The figure shows three views and two pictorial views of one solid part (mm, origin at its lowest corner). Answer the questions. A direction names the side the tool comes from. Coordinates: 2 decimals unless noted, no trailing zeros. Order: outer loops, then holes, each group sorted by start corner. A loop starts at its lowest first (then second) coordinate and runs counter-clockwise, first axis right, second up. Notation, with made-up numbers: (30, 45.5) -> (78, 45.5) arc R3 cw to (78, 49.5) -> close; hole circle Ø4 at (47.5, 79). An arc over 180 degrees is marked (long way). Write item = value, one per line.
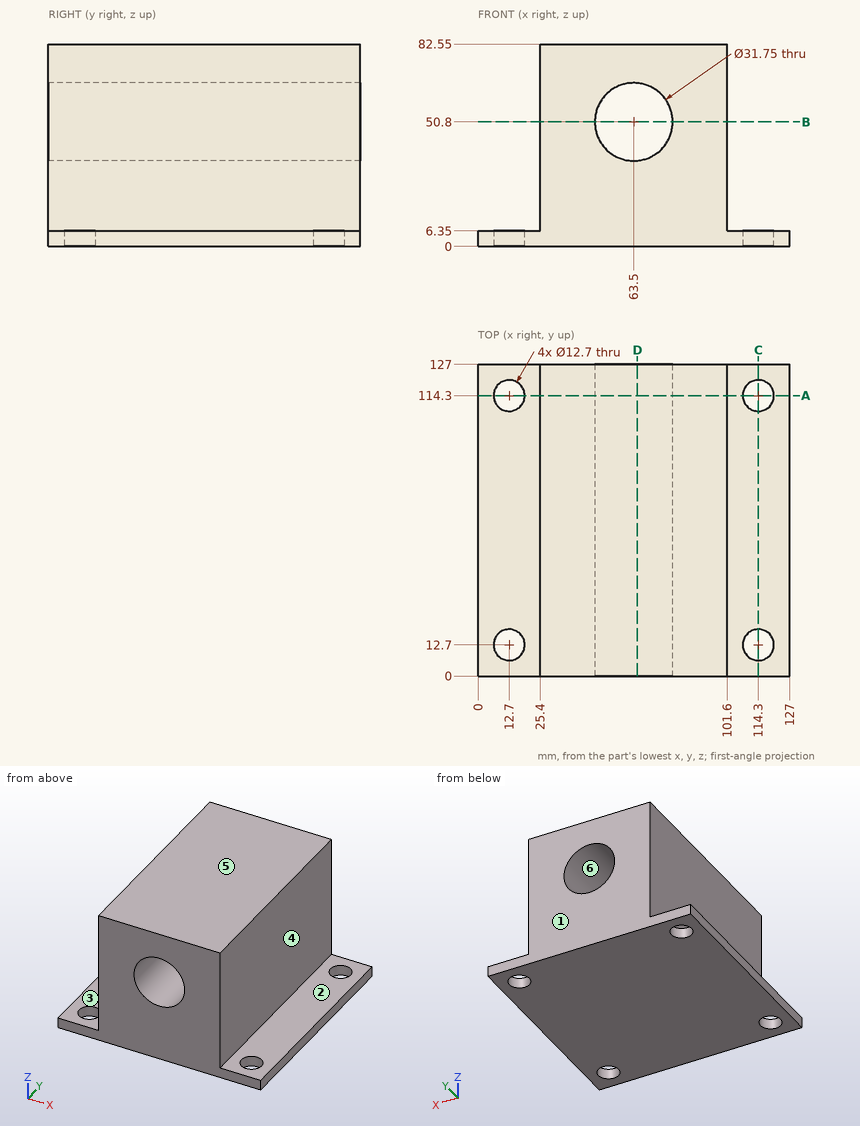
Q1. The mould has two halves that part along X. Classify the marked faces 4, 5 and 6: released by +X, released by -X, zero draft, split by the parting line, or undercut.
The answers:
face_4 = released by +X
face_5 = zero draft
face_6 = undercut
Q2. Section C-C, the plane x = 114.3 is taken. Give the vertices of the cut face in (y, z).
The answers:
outline = (0, 0) -> (6.35, 0) -> (6.35, 6.35) -> (0, 6.35) -> close; (19.05, 0) -> (107.95, 0) -> (107.95, 6.35) -> (19.05, 6.35) -> close; (120.65, 0) -> (127, 0) -> (127, 6.35) -> (120.65, 6.35) -> close
Q3. Section A-A, the plane y = 114.3 is taken. Give the vertices of the cut face in (x, z) (3 decimals).
The answers:
outline = (0, 0) -> (6.35, 0) -> (6.35, 6.35) -> (0, 6.35) -> close; (19.05, 0) -> (107.95, 0) -> (107.95, 6.35) -> (101.6, 6.35) -> (101.6, 82.55) -> (25.4, 82.55) -> (25.4, 6.35) -> (19.05, 6.35) -> close; (120.65, 0) -> (127, 0) -> (127, 6.35) -> (120.65, 6.35) -> close; hole circle Ø31.75 at (63.5, 50.8)
Q4. Section D-D, the plane x = 65 is taken. Give the vertices of the cut face in (y, z).
The answers:
outline = (0, 0) -> (127, 0) -> (127, 35) -> (0, 35) -> close; (0, 66.6) -> (127, 66.6) -> (127, 82.55) -> (0, 82.55) -> close
Q5. Each of these flat-tipped pins is pushed along its axis until it touches: pin 1 Ø3 at (y, z) = (52, 26) entering from +X; pin 2 Ø20.5 at (x, y) = (10.5, 84) entering from +Z; pin 3 Ø3 at (x, y) = (113.5, 96) entering from +Z. Where does it stop, or does it pass through?
The answers:
pin_1 = 101.6
pin_2 = 6.35
pin_3 = 6.35
Q6. Find the intervals of material crossed by line 1 along Y through (x, z) = (12.7, 1.75); line 2 along X through (y, z) = (12, 2); line 3 along X through (y, z) = (59, 50), in increasing order.
The answers:
line_1 = 0 to 6.35, 19.05 to 107.95, 120.65 to 127
line_2 = 0 to 6.39, 19.01 to 107.99, 120.61 to 127
line_3 = 25.4 to 47.65, 79.35 to 101.6
Q7. A tool of negligible diameter and unlimited length cuts with its end or side. For the marked faces 1, 2 and 3, from which of +Z, -Z, +X, -X, +Y, -Y can it reach the whole face along a straight path? Write none if from no direction.
The answers:
face_1 = +Z, -Z, +X, -X, +Y
face_2 = +Z, +X, +Y, -Y
face_3 = +Z, -X, +Y, -Y
Q8. Section B-B, the plane z = 50.8 is taken. Give the vertices of the cut face in (x, y) (3 decimals).
The answers:
outline = (25.4, 0) -> (47.625, 0) -> (47.625, 127) -> (25.4, 127) -> close; (79.375, 0) -> (101.6, 0) -> (101.6, 127) -> (79.375, 127) -> close
